from build123d import *

# Parameters (mm, degrees)
F0_W     = 34.925
F0_H     = 19.05
F0_R     = 0.79375
F1_DEPTH = 1.5875
F2_DEPTH = 3.175
F3_R     = 9.525


with BuildPart() as f1:
    # F0 (on Top) → F1 (new body, symmetric)
    with BuildSketch(Plane.XY):
        Rectangle(F0_W, F0_H)
        with Locations((-7.9375, 0.635)):
            Circle(F0_R, mode=Mode.SUBTRACT)
        with Locations((7.9375, 0.635)):
            Circle(F0_R, mode=Mode.SUBTRACT)
        with Locations((-7.9375, 0.635)):
            Circle(F0_R)
        with Locations((7.9375, 0.635)):
            Circle(F0_R)
    extrude(amount=F1_DEPTH, both=True)

    # F0 (on Top) → F2 (join)
    with BuildSketch(Plane.XY):
        with Locations((-7.9375, 0.635)):
            Circle(F0_R)
        with Locations((7.9375, 0.635)):
            Circle(F0_R)
    extrude(amount=F2_DEPTH)

    # F3
    f3_edges = [f1.edges().sort_by_distance(p)[0] for p in [
        (17.4625, -9.525, 0),
        (-17.4625, -9.525, 0),
    ]]
    fillet(f3_edges, radius=F3_R)


solid = f1.part
Build history of the part. All positions in model axes, mm. A direction names the side the tool comes from. Round coordinates to 2 decimals unless told otherwise and drop trailing zeros. Write each loop counter-clockwise with the first axis right and the second up, starting at its lowest first coordinate (ties: lowest second). Pieces come first, ordered by that corner, then holes. Notation, with made-up numbers: M 16,-9 L 27,-9 A16 ccw 27,22 Z; hole C -11,-37 d6. An arc over 180 degrees is marked long. Answer in a Markdown table with one row per item.
1. Which spindle directions (+Z, -Z, +X, -X, +Y, -Y) get a long thin tool onto all of the face, cutting with end or side? Do faces 1 (the face through (14.598, -6.809, 0.022)), 2 (the face through (-8.73, 0.67, 2.37)). Say none if no direction does.
Geometry check:
| item | result |
|---|---|
| face 1 | +Z, -Z, +X, -Y |
| face 2 | +Z |
2. Saw through at C-C (y = 3). List the corners of the cut face in (x, z), and give its area (3 significant figures).
Geometry check:
| item | result |
|---|---|
| outline | M -17.46,-1.59 L 17.46,-1.59 L 17.46,1.59 L -17.46,1.59 Z |
| area | 111 mm2 |
3. Mould opens along X. For faces 3 (the face through (8, 1, 3.175)), 4 (the face through (-17.462, 5, 0)), 5 (the face through (7.77, -0.14, 2.37)) say: +X half, -X half, draft (parallel to the pull), parting line (faces both ways), or undercut.
Geometry check:
| item | result |
|---|---|
| face 3 | draft |
| face 4 | -X half |
| face 5 | undercut |
4. Saw through at A-A (x = -4.5). List the corners of the cut face in (y, z) (1 decimal).
Geometry check:
| item | result |
|---|---|
| outline | M -9.5,-1.6 L 9.5,-1.6 L 9.5,1.6 L -9.5,1.6 Z |
5. Flat gauge pins, fed straight in: P1, Ø1.5, axis at y = 5, z = 2.5, coming from the -X side; P2, Ø3, axis at x = 5.5, y = -6.5, coming from the +Z side. Where does each tip first touch, or does it go through?
Geometry check:
| item | result |
|---|---|
| P1 | through |
| P2 | z = 1.59 |
6. Probe L1, parallel to Z at x = 6, y = -0.5; L2, parallel to Y at x = 8, z = 2.3; L3, parallel to Y at x = -15.5, z = 0.25 (3 decimals). List the from-to ranges inside material, lowest first. Write a range as [from, to].
Geometry check:
| item | result |
|---|---|
| L1 | [-1.59, 1.59] |
| L2 | [-0.16, 1.43] |
| L3 | [-5.791, 9.525] |
7. Saw through at D-D (z = 2.8). List the corners of the cut face in (x, y) (1 decimal).
Geometry check:
| item | result |
|---|---|
| outline | C -7.9,0.6 d1.6; C 7.9,0.6 d1.6 |
